Read the model definition and answer for the solid it produces. Units are mm, in the model's axes. Face numbers are marked on the shaded views. A direction names the side the tool comes from. Coordinates: 2 decimals unless noted, no trailing zeros. Write each loop counter-clockwise with the first axis right and the second up, starting at its lowest first coordinate (ties: lowest second). Pieces come first, ordered by that corner, then holes. Notation, with made-up numbers: (39.25, 6) -> (49.25, 6) arc R25 cw to (49.25, 33) -> close; hole circle Ø11 at (83.25, -8). An arc over 180 degrees is marked (long way). Answer in a Markdown table with one row per item. Add a question column.
Item 1: Given pin 1 Ø1.5 at (x, y) = (31.5, 21.5) entering from +Z; pin 2 Ø3 at (y, z) = (-17, 17.5) entering from -X; pin 3 Ø1 at (y, z) = (-2.5, 34.5) entering from -X; pin 4 Ø16 at (x, y) = (0, 0) entering from -Z, each flat-ended and moving along its own axis, determine where each tip first touches the part or whether it passes through.
Item 2: Section C-C on z = 29 is taken. Write down the section's boundary in (x, y), then the cut area to 3 significant figures.
Item 3: Which of the six approach directions +Z, -Z, +X, -X, +Y, -Y give full straight-line access (tool end or side, diameter ignored) to the marked faces 1, 2 and 3?
Item 4: Straight lines are drawn through the part: line 1 (Y direction, x = 0, z = 65); line 2 (Y direction, x = 0, z = 27); line 3 (Z direction, x = 8, y = -25.5). For each, find the intervals that lie inside material, in ascending order. Write a range as from..to.
Item 5: For a pull along X with two mould halves and no side action, classify the marked faces 4, 5 and 6 as +X half, -X half, draft (parallel to the pull), parting line (faces both ways), or undercut.
Item 6: Section D-D on z = 59 is taken. Write down the section's boundary in (x, y).
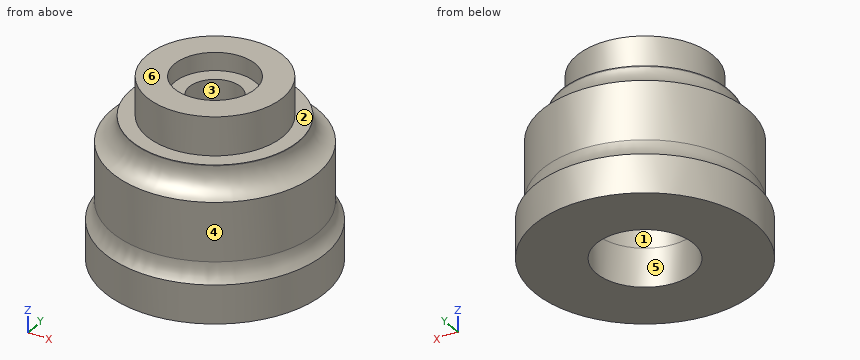
```python
from build123d import *

# Parameters (mm, degrees)
SKETCH_1_R          = 43
SKETCH_1_R_2        = 18.9
EXTRUDE_1_DEPTH     = 15
SKETCH_3_R          = 40
SKETCH_3_R_2        = 19
EXTRUDE_2_DEPTH     = 30
SKETCH_7_R          = 32.5
SKETCH_7_R_2        = 10
EXTRUDE_3_DEPTH     = 10
FILLET_3_R          = 10
SKETCH_9_R          = 16
SKETCH_9_R_2        = 10
EXTRUDE_6_DEPTH     = 7
SKETCH_10_R         = 26.5
SKETCH_10_R_2       = 10
EXTRUDE_7_DEPTH     = 15
SKETCH_12_R         = 15.75
CUT_EXTRUDE_8_DEPTH = 7
FILLET_4_R          = 10


with BuildPart() as part:
    # Sketch 1 → Extrude 1 (new body)
    with BuildSketch(Plane.XY):
        Circle(SKETCH_1_R)
        Circle(SKETCH_1_R_2, mode=Mode.SUBTRACT)
    extrude(amount=EXTRUDE_1_DEPTH)

    # Sketch 3 → Extrude 2 (add)
    with BuildSketch(Plane.XY.offset(15)):
        Circle(SKETCH_3_R)
        Circle(SKETCH_3_R_2, mode=Mode.SUBTRACT)
    extrude(amount=EXTRUDE_2_DEPTH)

    # Sketch 7 → Extrude 3 (add)
    with BuildSketch(Plane.XY.offset(45)):
        Circle(SKETCH_7_R)
        Circle(SKETCH_7_R_2, mode=Mode.SUBTRACT)
    extrude(amount=EXTRUDE_3_DEPTH)

    # Fillet 3
    # the kernel refuses this fillet: 10 mm, written as the material it adds along each edge
    with BuildSketch(Plane(origin=(0, 0, 15), x_dir=(1, 0, 0), z_dir=(0, -1, 0))) as fillet_3_piece_1:
        with BuildLine():
            CenterArc((50, 7.141428429), FILLET_3_R, 180, 45.572995999)
            Line((40, 7.141428429), (39.8, 7.141428429))
            Line((39.8, 7.141428429), (39.8, 0))
            Line((39.8, 0), (40, -0.2))
            ThreePointArc((40, -0.2), (41.5, -0.2), (42.86, -0.142828569))
            Line((42.86, -0.142828569), (43, 0))
        make_face()
    revolve(axis=Axis((0, 0, 15), (0, 0, 1)))



with BuildPart() as body_2:
    # Sketch 9 → Extrude 6 (new body)
    with BuildSketch(Plane.XY.offset(48)):
        Circle(SKETCH_9_R)
        Circle(SKETCH_9_R_2, mode=Mode.SUBTRACT)
    extrude(amount=EXTRUDE_6_DEPTH)


with BuildPart() as part_1:
    add(part.part)

    add(body_2.part)  # Extrude 7 merges body 2
    # Sketch 10 → Extrude 7 (add)
    with BuildSketch(Plane.XY.offset(55)):
        Circle(SKETCH_10_R)
        Circle(SKETCH_10_R_2, mode=Mode.SUBTRACT)
    extrude(amount=EXTRUDE_7_DEPTH)

    # Sketch 12 → Cut-Extrude 8 (cut)
    with BuildSketch(Plane.XY.offset(70)):
        Circle(SKETCH_12_R)
    extrude(amount=-CUT_EXTRUDE_8_DEPTH, mode=Mode.SUBTRACT)

    # Fillet 4
    # the kernel refuses this fillet: 10 mm, written as the material it adds along each edge
    with BuildSketch(Plane(origin=(0, 0, 45), x_dir=(1, 0, 0), z_dir=(0, -1, 0))) as fillet_4_piece_1:
        with BuildLine():
            CenterArc((42.5, 9.682458366), FILLET_4_R, 180, 75.522487814)
            Line((32.5, 9.682458366), (32.3, 9.682458366))
            Line((32.3, 9.682458366), (32.3, 0))
            Line((32.3, 0), (32.5, -0.2))
            ThreePointArc((32.5, -0.2), (36.25, -0.2), (39.95, -0.193649167))
            Line((39.95, -0.193649167), (40, 0))
        make_face()
    revolve(axis=Axis((0, 0, 45), (0, 0, 1)))


solid = part_1.part
```
Results below:
| question | item | result |
|---|---|---|
| 1 | pin 1 | stops at z = 46.09 |
| 1 | pin 2 | stops at x = -38.68 |
| 1 | pin 3 | stops at x = -39.95 |
| 1 | pin 4 | passes through |
| 2 | outline | circle Ø80 at (0, 0); hole circle Ø38 at (0, 0) |
| 2 | area | 3,890 mm2 |
| 3 | face 1 | none |
| 3 | face 2 | +Z |
| 3 | face 3 | +Z, -Z |
| 4 | line 1 | y = -26.5..-15.75, 15.75..26.5 |
| 4 | line 2 | y = -40..-19, 19..40 |
| 4 | line 3 | z = 0..55 |
| 5 | face 4 | parting line |
| 5 | face 5 | undercut |
| 5 | face 6 | draft |
| 6 | outline | circle Ø53 at (0, 0); hole circle Ø20 at (0, 0) |
